Verification items for the finished model (mm, model axes). A direction names the side the tool comes from. Give positions to 0.01 mm unless a question says otherwise; leave off trailing zeros. Order: outer loops, then holes, each group sorted by start corner. A loop starts at its lowest first (then second) coordinate and runs counter-clockwise, first axis right, second up. Notation, with made-up numbers: (52, 59) -> (84, 59) arc R30 ccw to (84, 91) -> close; hole circle Ø1 at (28, 50.25). An arc over 180 degrees is marked (long way). Return JSON: item names as keys, results as strings. Group by question number.
(1) Cross-section at A-A on y = 5. Enter the section's corners in (x, z).
(2) Cross-section at B-B on z = 175.5. Enter the section's corners in (x, y), then the cut area to 3 significant figures.
(3) Thickness scan on line 1 along X through (y, z) = (60, 193.5); line 2 along Z through (x, y) = (-12.5, 101); line 3 along Z through (x, y) = (0.5, 82.5). Record the ranges inside material, lowest first.
(4) Tool access check on faces 1 (the face through (-3, 104.91, 311)), 2 (the face through (0, 55, 150)), 3 (the face through (-3, 105.77, 311)), 4 (the face through (1.57, 55, 150)). Record the directions out of +Z, -Z, +X, -X, +Y, -Y that give a thin tool (end or side, any length) a straight path to the whole face; none if there is none.
(5) Depth check by flat-ended pin: pin 1 Ø9 at (x, z) = (-7, 314) entering from -Y; pin 2 Ø3 at (y, z) = (30, 110.5) entering from +X; pin 3 Ø6 at (y, z) = (67, 124) entering from -X. Enter the tip coordinate at first touch or a pass-through.
from build123d import *

# Parameters (mm, degrees)
SKETCH1_W           = 1.57
SKETCH1_H           = 111.15
PCB_DEPTH           = 304.8
BOSS_EXTRUDE2_DEPTH = 0.86
CUT_EXTRUDE1_REACH  = 327.615
CUT_EXTRUDE2_REACH  = 327.615
FILLET2_R           = 1.27
FILLET1_R           = 1.91
SKETCH8_W           = 19.05
SKETCH8_H           = 0.86
BOSS_EXTRUDE4_DEPTH = 12.29
CUT_EXTRUDE3_REACH  = 341.707


with BuildPart() as part:
    # Sketch1 → pcb (new body)
    with BuildSketch(Plane.XY):
        with Locations((0.785, 55.575)):
            Rectangle(SKETCH1_W, SKETCH1_H)
    extrude(amount=PCB_DEPTH)

    # mounting-slot → Boss-Extrude2 (add)
    with BuildSketch(Plane.XY.offset(304.8)):
        Polygon((-15.58, 104.91), (2.84, 104.91), (6.01, 104.91), (6.01, 100.35), (2.84, 100.35), (2.84, -3.73), (-1.27, -7.84), (-1.27, -15.11), (-11.46, -15.11), (-11.46, -7.84), (-15.58, -3.72), align=None)
    extrude(amount=BOSS_EXTRUDE2_DEPTH)

    # Sketch5 → Cut-Extrude1 (cut, up to next)
    with BuildSketch(Plane.XY.offset(305.66), mode=Mode.PRIVATE) as cut_extrude1_sk1:
        Polygon((-15.58, 99.29), (-13.04, 101.83), (-13.04, 104.91), (-15.58, 104.91), align=None)
    cut_extrude1_tool1 = extrude(cut_extrude1_sk1.sketch, amount=-CUT_EXTRUDE1_REACH, mode=Mode.PRIVATE) & part.part
    add(cut_extrude1_tool1.solids().sort_by_distance((-14.433594, 102.673203, 305.66))[0], mode=Mode.SUBTRACT)

    # Sketch7 → Cut-Extrude2 (cut, up to next)
    with BuildSketch(Plane.XY.offset(305.66), mode=Mode.PRIVATE) as cut_extrude2_sk1:
        Polygon((6.01, 101.99), (4.37, 100.35), (6.01, 100.35), align=None)
    cut_extrude2_tool1 = extrude(cut_extrude2_sk1.sketch, amount=-CUT_EXTRUDE2_REACH, mode=Mode.PRIVATE) & part.part
    add(cut_extrude2_tool1.solids().sort_by_distance((5.463333, 100.896667, 305.66))[0], mode=Mode.SUBTRACT)

    # Fillet2
    fillet2_edges = [part.edges().sort_by_distance(p)[0] for p in [
        (4.37, 100.35, 305.23),
    ]]
    fillet(fillet2_edges, radius=FILLET2_R)

    # Fillet1
    fillet1_edges = [part.edges().sort_by_distance(p)[0] for p in [
        (-11.46, -15.11, 305.23),
        (-1.27, -15.11, 305.23),
    ]]
    fillet(fillet1_edges, radius=FILLET1_R)

    # Sketch8 → Boss-Extrude4 (add)
    with BuildSketch(Plane(origin=(0, 0, 304.8), x_dir=(-1, 0, 0), z_dir=(0, 0, -1))):
        with Locations((3.515, 105.34)):
            Rectangle(SKETCH8_W, SKETCH8_H)
    extrude(amount=-BOSS_EXTRUDE4_DEPTH)

    # Sketch9 → Cut-Extrude3 (cut, up to next)
    with BuildSketch(Plane(origin=(0, 105.77, 0), x_dir=(1, 0, 0), z_dir=(0, 1, 0)), mode=Mode.PRIVATE) as cut_extrude3_sk1:
        Polygon((-9.23, -317.09), (-5.42, -313.28), (-5.42, -312.9), (-2.37, -312.9), (-2.37, -313.28), (1.44, -317.09), align=None)
    cut_extrude3_tool1 = extrude(cut_extrude3_sk1.sketch, amount=-CUT_EXTRUDE3_REACH, mode=Mode.PRIVATE) & part.part
    # Sketch9 → Cut-Extrude3 (cut, up to next)
    with BuildSketch(Plane(origin=(0, 105.77, 0), x_dir=(1, 0, 0), z_dir=(0, 1, 0)), mode=Mode.PRIVATE) as cut_extrude3_sk2:
        with BuildLine():
            Line((6.01, -308.53), (3.465, -308.53))
            ThreePointArc((3.465, -308.53), (1.255, -310.74), (3.465, -312.95))
            Line((3.465, -312.95), (6.01, -312.95))
            Line((6.01, -312.95), (6.01, -308.53))
        make_face()
    cut_extrude3_tool2 = extrude(cut_extrude3_sk2.sketch, amount=-CUT_EXTRUDE3_REACH, mode=Mode.PRIVATE) & part.part
    add(cut_extrude3_tool1.solids().sort_by_distance((-3.895, 105.77, 315.433744))[0], mode=Mode.SUBTRACT)
    add(cut_extrude3_tool2.solids().sort_by_distance((3.841216, 105.77, 310.74))[0], mode=Mode.SUBTRACT)


solid = part.part
Verdict:
{
 "1": {"outline": "(-15.58, 304.8) -> (0, 304.8) -> (0, 0) -> (1.57, 0) -> (1.57, 304.8) -> (2.84, 304.8) -> (2.84, 305.66) -> (-15.58, 305.66) -> close"},
 "2": {"outline": "(0, 0) -> (1.57, 0) -> (1.57, 111.15) -> (0, 111.15) -> close", "area": "175 mm²"},
 "3": {"line 1": "0 to 1.57", "line 2": "304.8 to 305.66", "line 3": "0 to 305.66"},
 "4": {"face 1": "+Z, +X, -X, -Y", "face 2": "-Z, -X, +Y, -Y", "face 3": "+Z, +X, -X, +Y", "face 4": "-Z, +X, +Y, -Y"},
 "5": {"pin 1": "y = 104.91", "pin 2": "x = 1.57", "pin 3": "x = 0"}
}
